Read the model definition and answer for the solid it produces. Units are mm, in the model's axes. Face numbers are marked on the shaded views. A direction names the side the tool comes from. Round coordinates to 2 decimals unless told otherwise and drop trailing zeros. One line per item, written item: value. Start each with the question number.
1. For the marked faces 4, 5 and 6, determine the directions among +Z, -Z, +X, -X, +Y, -Y from which every point of the face is accessible in a straight line to the end or side of a thin tool.
2. Section A-A (x = 17) is taken. State how many separate pieces and enclosed holes the cut face has, then the cut area to 3 significant figures.
3. The mould has two halves that part along X. Classify the marked faces 1, 2 and 3: released by +X, released by -X, zero draft, split by the parting line, or undercut.
4. Consider line 1 (Y direction, x = 16, z = 3); line 2 (Y direction, x = 16, z = 6); line 3 (Y direction, x = 15, z = 6). Determine where each line is inside the solid, lowest interval first.
5. Flat-ended cylindrical pins translate along their axes: pin 1 Ø0.8 at (y, z) = (-14.5, 5.5) entering from -X; pin 2 Ø4 at (x, y) = (5, 2.5) entering from -Z; pin 3 Ø1.6 at (x, z) = (-7.5, 6.5) entering from +Y; pin 4 Ø2.5 at (x, y) = (16, -7.5) entering from +Z. Find the tip coordinate at first contact, or state that the pin passes through.
from build123d import *

# Parameters (mm, degrees)
BOSS_EXTRUDE1_DEPTH = 12
FILLET1_R           = 5
SKETCH5_W           = 10.5
SKETCH5_H           = 6
CUT_EXTRUDE3_DEPTH  = 37.349002737
SKETCH6_W           = 5
SKETCH6_H           = 2
BOSS_EXTRUDE2_DEPTH = 5
FILLET2_R           = 2.5
FILLET3_R           = 2.5
SKETCH3_R           = 1.65
CUT_EXTRUDE4_DEPTH  = 31.352100461
SKETCH8_R           = 0.75
CUT_EXTRUDE7_DEPTH  = 51.387859352
SKETCH9_R           = 0.75
CUT_EXTRUDE9_DEPTH  = 23.34523506


with BuildPart() as part:
    # Sketch2 → Boss-Extrude1 (new body)
    with BuildSketch(Plane.XY):
        with BuildLine():
            Line((-16, 0), (16, 0))
            ThreePointArc((16, 0), (23.5, -7.5), (16, -15))
            Line((16, -15), (-16, -15))
            ThreePointArc((-16, -15), (-23.5, -7.5), (-16, 0))
        make_face()
    extrude(amount=BOSS_EXTRUDE1_DEPTH)

    # Fillet1
    fillet1_edges = [part.edges().sort_by_distance(p)[0] for p in [
        (-23.5, -7.5, 12),
        (0, -15, 12),
        (23.5, -7.5, 12),
        (0, -15, 0),
        (-23.5, -7.5, 0),
        (0, 0, 0),
        (23.5, -7.5, 0),
        (0, 0, 12),
    ]]
    fillet(fillet1_edges, radius=FILLET1_R)

    # Sketch5 → Cut-Extrude3 (cut, through all)
    with BuildSketch(Plane(origin=(0, -25, 0), x_dir=(-1, 0, 0), z_dir=(0, -1, 0))):
        with Locations((18.25, -6)):
            Rectangle(SKETCH5_W, SKETCH5_H)
    extrude(amount=-CUT_EXTRUDE3_DEPTH, mode=Mode.SUBTRACT)

    # Sketch6 → Boss-Extrude2 (add)
    with BuildSketch(Plane(origin=(0, 0, 0), x_dir=(1, 0, 0), z_dir=(0, 1, 0))):
        with Locations((5.5, -6)):
            Rectangle(SKETCH6_W, SKETCH6_H)
    extrude(amount=BOSS_EXTRUDE2_DEPTH)

    # Fillet2
    fillet2_edges = [part.edges().sort_by_distance(p)[0] for p in [
        (8, 5, 6),
        (3, 5, 6),
    ]]
    fillet(fillet2_edges, radius=FILLET2_R - 0.0001)  # a hair under: the kernel refuses the full size

    # Fillet3
    fillet3_edges = [part.edges().sort_by_distance(p)[0] for p in [
        (3, 0, 6),
        (8, 0, 6),
    ]]
    fillet(fillet3_edges, radius=FILLET3_R)

    # Sketch3 → Cut-Extrude4 (cut, through all)
    with BuildSketch(Plane.XY.offset(12)):
        with Locations((-16, -7.5)):
            Circle(SKETCH3_R)
        with Locations((16, -7.5)):
            Circle(SKETCH3_R)
    extrude(amount=-CUT_EXTRUDE4_DEPTH, mode=Mode.SUBTRACT)

    # Sketch8 → Cut-Extrude7 (cut, through all)
    with BuildSketch(Plane(origin=(23.5, 0, 0), x_dir=(0, 0, -1), z_dir=(1, 0, 0))):
        with Locations((-6, -4)):
            Circle(SKETCH8_R)
    extrude(amount=-CUT_EXTRUDE7_DEPTH, mode=Mode.SUBTRACT)

    # Sketch9 → Cut-Extrude9 (cut, along a direction that is not the sketch's normal)
    with BuildSketch(Plane.ZY.offset(13)):
        with Locations((6, -11)):
            Circle(SKETCH9_R)
    extrude(amount=-CUT_EXTRUDE9_DEPTH, dir=(-0.9852117548196745, 0.17134117475124766, 0), mode=Mode.SUBTRACT)


solid = part.part
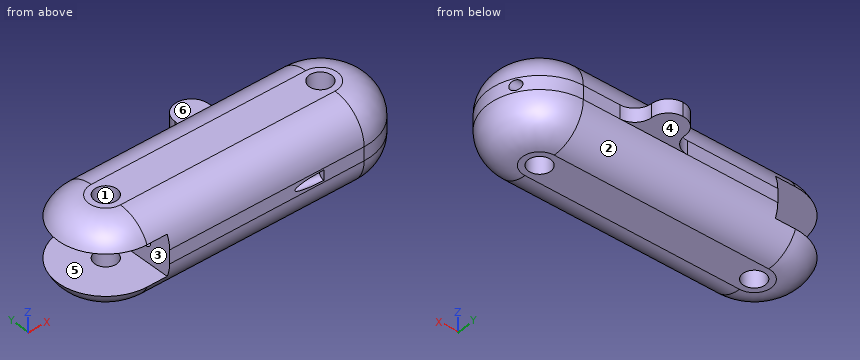
Answer:
1. face 4: -Z, +X, -X, +Y
1. face 5: -X, +Y, -Y
1. face 6: +Z, +X, -X, +Y
2. separate pieces: 2
2. enclosed holes: 1
2. area: 123 mm^2
3. face 1: undercut
3. face 2: zero draft
3. face 3: released by -X
4. line 1: -14.58 to -9.15, -5.85 to -0.42
4. line 2: -15 to -9.15, -5.85 to -4.75, -3.25 to 0
4. line 3: -15 to -8.81, -6.19 to -4.75, -3.25 to 0
5. pin 1: x = -13
5. pin 2: z = 5
5. pin 3: y = 0
5. pin 4: through
